Here's how the part is built. I have some questions about the finished solid (model axes, mm). A direction names the side the tool comes from. Give positions to 0.01 mm unless a question says otherwise; leave off trailing zeros. Loops run counter-clockwise (first coordinate to the right, second up) from the corner with the lowest first, then second, coordinate; pieces in that order, holes last.
Q1. I need wall thicknesses on probe 1 along X at (y, z) = (39.5, 2.75); probe 2 along X at (y, z) = (26.5, -3.75); probe 3 along X at (y, z) = (4.5, 11.75). Which ranges of each line are inside material? Lowest first, please.
Q2. Suppose I cut it at A-A (z = 12). List the corners of the cut face in (x, y) for me.
Q3. I'm going to push flat-ended pins straight in: P1, Ø2, axis at x = -18.5, z = 10, coming from the +Y side; P2, Ø4, axis at x = -9.5, z = -9, coming from the +Y side; P3, Ø4, axis at x = -6.5, y = 28, coming from the -Z side. Where does each tip first touch, or does it pass through?
Q4. For faces 1 (the face through (4, 15, -6)), 2 (the face through (-10, 26, 3)), 3 (the face through (20, 50, 0)), which set-ups out of +Z, -Z, +X, -X, +Y, -Y let a thin tool reach every point of the face, with its end or its side?
Q5. Suppose I cut it at D-D (x = 0). List the corners of the cut face in (y, z) for me, and give its area (3 significant figures).
Q6. Suppose I cut it at C-C (y = 29). List the corners of the cut face in (x, z) for me, and give its area (3 significant figures).
Q7. Thinking about a two-plate mould opening in X: for faces 4 (the face through (-24.43, 6.4, 10.23)), 5 (the face through (0, 57, 0)), 6 (the face through (-22, 30, 0)), which applies, pulls with the +X half, pulls with the -X half, needs draft (parallel to the pull), parting line crosses it, or undercut?
Q8. Suppose I cut it at B-B (x = 20). List the corners of the cut face in (y, z) for me.
```python
from build123d import *

# Parameters (mm, degrees)
SKETCH2_W                      = 50
SKETCH2_H                      = 30
BOSS_EXTRUDE1_DEPTH            = 7
SKETCH3_W                      = 50
SKETCH3_H                      = 16
BOSS_EXTRUDE2_DEPTH            = 50
SKETCH5_W                      = 30
SKETCH5_H                      = 6
CUT_EXTRUDE1_DEPTH             = 52
CUT_EXTRUDE3_REACH             = 68.355
CUT_EXTRUDE3_DIRECTION_2_REACH = 68.355
CUT_EXTRUDE4_REACH             = 68.355
CUT_EXTRUDE4_DIRECTION_2_REACH = 68.355
CUT_EXTRUDE5_REACH             = 68.355
FILLET1_R                      = 2
FILLET2_R                      = 0.5


with BuildPart() as part:
    # Sketch2 → Boss-Extrude1 (new body)
    with BuildSketch(Plane(origin=(0, 0, 0), x_dir=(1, 0, 0), z_dir=(0, 1, 0))):
        Rectangle(SKETCH2_W, SKETCH2_H)
    extrude(amount=BOSS_EXTRUDE1_DEPTH)

    # Sketch3 → Boss-Extrude2 (add)
    with BuildSketch(Plane(origin=(0, 7, 0), x_dir=(1, 0, 0), z_dir=(0, 1, 0))):
        Rectangle(SKETCH3_W, SKETCH3_H)
    extrude(amount=BOSS_EXTRUDE2_DEPTH)

    # Sketch5 → Cut-Extrude1 (cut)
    with BuildSketch(Plane.XZ):
        Rectangle(SKETCH5_W, SKETCH5_H)
    extrude(amount=-CUT_EXTRUDE1_DEPTH, mode=Mode.SUBTRACT)

    # Sketch4 → Cut-Extrude3 (cut, up to next)
    with BuildSketch(Plane.XY.offset(8), mode=Mode.PRIVATE) as cut_extrude3_sk1:
        with BuildLine():
            Line((-9.5, 15), (-9.5, 37))
            ThreePointArc((-9.5, 37), (0, 46.5), (9.5, 37))
            Line((9.5, 37), (9.5, 15))
            Line((9.5, 15), (9.5, 0))
            Line((9.5, 0), (-9.5, 0))
            Line((-9.5, 0), (-9.5, 15))
        make_face()
    cut_extrude3_tool1 = extrude(cut_extrude3_sk1.sketch, amount=-CUT_EXTRUDE3_REACH, mode=Mode.PRIVATE) & part.part
    add(cut_extrude3_tool1.solids().sort_by_distance((0, 22.281201, 8))[0], mode=Mode.SUBTRACT)

    # Sketch4 → Cut-Extrude3 direction 2 (cut, up to next)
    with BuildSketch(Plane.XY.offset(8), mode=Mode.PRIVATE) as cut_extrude3_direction_2_sk1:
        with BuildLine():
            Line((-9.5, 15), (-9.5, 37))
            ThreePointArc((-9.5, 37), (0, 46.5), (9.5, 37))
            Line((9.5, 37), (9.5, 15))
            Line((9.5, 15), (9.5, 0))
            Line((9.5, 0), (-9.5, 0))
            Line((-9.5, 0), (-9.5, 15))
        make_face()
    cut_extrude3_direction_2_tool1 = extrude(cut_extrude3_direction_2_sk1.sketch, amount=CUT_EXTRUDE3_DIRECTION_2_REACH, mode=Mode.PRIVATE) & part.part
    add(cut_extrude3_direction_2_tool1.solids().sort_by_distance((0, 22.281201, 8))[0], mode=Mode.SUBTRACT)

    # Sketch6 → Cut-Extrude4 (cut, up to next)
    with BuildSketch(Plane(origin=(0, 0, -8), x_dir=(-1, 0, 0), z_dir=(0, 0, -1)), mode=Mode.PRIVATE) as cut_extrude4_sk1:
        with BuildLine():
            Line((-4, 37), (-4, 0))
            Line((-4, 0), (4, 0))
            Line((4, 0), (4, 37))
            ThreePointArc((4, 37), (0, 41), (-4, 37))
        make_face()
    cut_extrude4_tool1 = extrude(cut_extrude4_sk1.sketch, amount=-CUT_EXTRUDE4_REACH, mode=Mode.PRIVATE) & part.part
    add(cut_extrude4_tool1.solids().sort_by_distance((0, 20.080724, -8))[0], mode=Mode.SUBTRACT)

    # Sketch6 → Cut-Extrude4 direction 2 (cut, up to next)
    with BuildSketch(Plane(origin=(0, 0, -8), x_dir=(-1, 0, 0), z_dir=(0, 0, -1)), mode=Mode.PRIVATE) as cut_extrude4_direction_2_sk1:
        with BuildLine():
            Line((-4, 37), (-4, 0))
            Line((-4, 0), (4, 0))
            Line((4, 0), (4, 37))
            ThreePointArc((4, 37), (0, 41), (-4, 37))
        make_face()
    cut_extrude4_direction_2_tool1 = extrude(cut_extrude4_direction_2_sk1.sketch, amount=CUT_EXTRUDE4_DIRECTION_2_REACH, mode=Mode.PRIVATE) & part.part
    add(cut_extrude4_direction_2_tool1.solids().sort_by_distance((0, 20.080724, -8))[0], mode=Mode.SUBTRACT)

    # Sketch8 → Cut-Extrude5 (cut, up to next)
    with BuildSketch(Plane.XY.offset(8), mode=Mode.PRIVATE) as cut_extrude5_sk1:
        with BuildLine():
            Line((-22, 48), (-22, 11))
            ThreePointArc((-22, 11), (-20, 9), (-18, 11))
            Line((-18, 11), (-18, 48))
            ThreePointArc((-18, 48), (-20, 50), (-22, 48))
        make_face()
    cut_extrude5_tool1 = extrude(cut_extrude5_sk1.sketch, amount=-CUT_EXTRUDE5_REACH, mode=Mode.PRIVATE) & part.part
    # Sketch8 → Cut-Extrude5 (cut, up to next)
    with BuildSketch(Plane.XY.offset(8), mode=Mode.PRIVATE) as cut_extrude5_sk2:
        with BuildLine():
            Line((18, 48), (18, 11))
            ThreePointArc((18, 11), (20, 9), (22, 11))
            Line((22, 11), (22, 48))
            ThreePointArc((22, 48), (20, 50), (18, 48))
        make_face()
    cut_extrude5_tool2 = extrude(cut_extrude5_sk2.sketch, amount=-CUT_EXTRUDE5_REACH, mode=Mode.PRIVATE) & part.part
    add(cut_extrude5_tool1.solids().sort_by_distance((-20, 29.5, 8))[0], mode=Mode.SUBTRACT)
    add(cut_extrude5_tool2.solids().sort_by_distance((20, 29.5, 8))[0], mode=Mode.SUBTRACT)

    # Fillet1
    fillet1_edges = [part.edges().sort_by_distance(p)[0] for p in [
        (25, 7, 11.5),
        (14.5, 7, -15),
        (-25, 7, 11.5),
        (25, 7, -11.5),
        (25, 32, -8),
        (-25, 32, -8),
        (-25, 32, 8),
        (25, 32, 8),
        (0, 57, -8),
        (-25, 57, 0),
        (0, 57, 8),
        (25, 57, 0),
        (-25, 7, -11.5),
        (17.25, 7, 15),
        (-14.5, 7, -15),
        (-17.25, 7, 15),
        (-25, 3.5, -15),
        (25, 3.5, -15),
        (25, 3.5, 15),
        (-25, 3.5, 15),
    ]]
    fillet(fillet1_edges, radius=FILLET1_R)

    # Fillet2
    fillet2_edges = [part.edges().sort_by_distance(p)[0] for p in [
        (-16.25, 7, 8),
        (13.5, 7, -8),
        (-24.526592034, 6.292097815, 7.292097815),
        (-24.526592034, 6.292097815, -7.292097815),
        (24.526592034, 6.292097815, 7.292097815),
        (24.526592034, 6.292097815, -7.292097815),
        (16.25, 7, 8),
        (-13.5, 7, -8),
    ]]
    fillet(fillet2_edges, radius=FILLET2_R)


solid = part.part
```
Solutions:
1. probe 1: x = -25 to -22, -18 to -15, 15 to 18, 22 to 25
1. probe 2: x = -25 to -22, -18 to -4, 4 to 18, 22 to 25
1. probe 3: x = -25 to -9.5, 9.5 to 25
2. outline: (-25, 0) - (-9.5, 0) - (-9.5, 7) - (-23, 7) arc R2 ccw to (-25, 5) - close; (9.5, 0) - (25, 0) - (25, 5) arc R2 ccw to (23, 7) - (9.5, 7) - close
3. P1: stops at y = 7
3. P2: stops at y = 56.73
3. P3: stops at z = -8
4. face 1: +Z, -Z, -Y
4. face 2: -Y
4. face 3: +Z, -Z
5. outline: (41, -8) - (55, -8) arc R2 ccw to (57, -6) - (57, 6) arc R2 ccw to (55, 8) - (46.5, 8) - (46.5, 3) - (52, 3) - (52, -3) - (41, -3) - close
5. area: 161 mm2
6. outline: (-25, -6) arc R2 ccw to (-23, -8) - (-22, -8) - (-22, 8) - (-23, 8) arc R2 ccw to (-25, 6) - close; (-18, -8) - (-4, -8) - (-4, -3) - (-15, -3) - (-15, 3) - (-9.5, 3) - (-9.5, 8) - (-18, 8) - close; (4, -8) - (18, -8) - (18, 8) - (9.5, 8) - (9.5, 3) - (15, 3) - (15, -3) - (4, -3) - close; (22, -8) - (23, -8) arc R2 ccw to (25, -6) - (25, 6) arc R2 ccw to (23, 8) - (22, 8) - close
6. area: 354 mm2
7. face 4: pulls with the -X half
7. face 5: needs draft
7. face 6: undercut
8. outline: (0, -15) - (5, -15) arc R2 ccw to (7, -13) - (7, -8.5) arc R0.5 cw to (7.5, -8) - (9, -8) - (9, 8) - (7.5, 8) arc R0.5 cw to (7, 8.5) - (7, 13) arc R2 ccw to (5, 15) - (0, 15) - close; (50, -8) - (55, -8) arc R2 ccw to (57, -6) - (57, 6) arc R2 ccw to (55, 8) - (50, 8) - close
